from build123d import *

# Parameters (mm, degrees)
F1_DEPTH = 50
F2_DEPTH = 13
F4_DEPTH = 74.001
F5_R     = 1.25
F6_DEPTH = 15
F7_W     = 3
F7_H     = 10
F8_DEPTH = 8
F7_R     = 1.75
F9_DEPTH = 25


with BuildPart() as f1:
    # F0 (on Top) → F1 (new body)
    with BuildSketch(Plane.XY):
        Polygon((-17.5, 12), (-17.5, 0), (0, 0), (17.5, 0), (17.5, 12), (13.5, 12), (13.5, 8), (-13.5, 8), (-13.5, 12), align=None)
    extrude(amount=-F1_DEPTH)

    # F0 (on Top) → F2 (join)
    with BuildSketch(Plane.XY):
        with BuildLine():
            Line((-37, 0), (-37, -8))
            ThreePointArc((-37, -8), (-30, -15), (-23, -8))
            Line((-23, -8), (-23, 0))
            Line((-23, 0), (-17.5, 0))
            Line((-17.5, 0), (-17.5, 12))
            Line((-17.5, 12), (-37, 4))
            Line((-37, 4), (-37, 0))
        make_face()
        with BuildLine():
            Line((17.5, 12), (17.5, 0))
            Line((17.5, 0), (23, 0))
            Line((23, 0), (23, -8))
            ThreePointArc((23, -8), (30, -15), (37, -8))
            Line((37, -8), (37, 0))
            Line((37, 0), (37, 4))
            Line((37, 4), (17.5, 12))
        make_face()
    extrude(amount=-F2_DEPTH)

    # F3 (on face) → F4 (cut, through all)
    with BuildSketch(Plane(origin=(-37, 0, 0), x_dir=(0, -1, 0), z_dir=(-1, 0, 0))):
        Polygon((8, -11.267949), (8, -13), (15, -13), (15, -7.226497), align=None)
        Polygon((5, -13), (8, -13), (8, -11.267949), align=None)
    extrude(amount=-F4_DEPTH, mode=Mode.SUBTRACT)

    # F5 (on face) → F6 (cut)
    with BuildSketch(Plane(origin=(0, -6.879165, -11.915064), x_dir=(1, 0, 0), z_dir=(0, -0.5, -0.866025))):
        with Locations((-30, 3.377132)):
            Circle(F5_R)
        with Locations((30, 3.377132)):
            Circle(F5_R)
    extrude(amount=-F6_DEPTH, mode=Mode.SUBTRACT)

    # F7 (on face) → F8 (join)
    with BuildSketch(Plane.XZ):
        with BuildLine():
            Line((17.03, 0), (7.03, 0))
            Line((7.03, 0), (7.03, -10))
            Line((7.03, -10), (8.197224, -10))
            ThreePointArc((8.197224, -10), (10, -9.5), (11.802776, -10))
            Line((11.802776, -10), (17.03, -10))
            Line((17.03, -10), (17.03, 0))
        make_face()
        with BuildLine():
            Line((6.39, -1.259825), (6.39, -1))
            Line((6.39, -1), (6.39, -0.740175))
            ThreePointArc((6.39, -0.740175), (6.352771, -0.641268), (6.259565, -0.591457))
            ThreePointArc((6.259565, -0.591457), (6.101938, -0.557612), (5.951798, -0.498876))
            ThreePointArc((5.951798, -0.498876), (5.724361, -0.294149), (5.64, 0))
            Line((5.64, 0), (-0.36, 0))
            ThreePointArc((-0.36, 0), (-0.444361, -0.294149), (-0.671798, -0.498876))
            ThreePointArc((-0.671798, -0.498876), (-0.821938, -0.557612), (-0.979565, -0.591457))
            ThreePointArc((-0.979565, -0.591457), (-1.072771, -0.641268), (-1.11, -0.740175))
            Line((-1.11, -0.740175), (-1.11, -1))
            Line((-1.11, -1), (-1.11, -1.259825))
            ThreePointArc((-1.11, -1.259825), (-1.072771, -1.358732), (-0.979565, -1.408543))
            ThreePointArc((-0.979565, -1.408543), (-0.821938, -1.442388), (-0.671798, -1.501124))
            ThreePointArc((-0.671798, -1.501124), (-0.444361, -1.705851), (-0.36, -2))
            ThreePointArc((-0.36, -2), (-0.444361, -2.294149), (-0.671798, -2.498876))
            ThreePointArc((-0.671798, -2.498876), (-0.821938, -2.557612), (-0.979565, -2.591457))
            ThreePointArc((-0.979565, -2.591457), (-1.072771, -2.641268), (-1.11, -2.740175))
            Line((-1.11, -2.740175), (-1.11, -3))
            Line((-1.11, -3), (-1.11, -3.259825))
            ThreePointArc((-1.11, -3.259825), (-1.072771, -3.358732), (-0.979565, -3.408543))
            ThreePointArc((-0.979565, -3.408543), (-0.821938, -3.442388), (-0.671798, -3.501124))
            ThreePointArc((-0.671798, -3.501124), (-0.444361, -3.705851), (-0.36, -4))
            ThreePointArc((-0.36, -4), (-0.444361, -4.294149), (-0.671798, -4.498876))
            ThreePointArc((-0.671798, -4.498876), (-0.821938, -4.557612), (-0.979565, -4.591457))
            ThreePointArc((-0.979565, -4.591457), (-1.072771, -4.641268), (-1.11, -4.740175))
            Line((-1.11, -4.740175), (-1.11, -5))
            Line((-1.11, -5), (-1.11, -5.259825))
            ThreePointArc((-1.11, -5.259825), (-1.072771, -5.358732), (-0.979565, -5.408543))
            ThreePointArc((-0.979565, -5.408543), (-0.821938, -5.442388), (-0.671798, -5.501124))
            ThreePointArc((-0.671798, -5.501124), (-0.444361, -5.705851), (-0.36, -6))
            ThreePointArc((-0.36, -6), (-0.444361, -6.294149), (-0.671798, -6.498876))
            ThreePointArc((-0.671798, -6.498876), (-0.821938, -6.557612), (-0.979565, -6.591457))
            ThreePointArc((-0.979565, -6.591457), (-1.072771, -6.641268), (-1.11, -6.740175))
            Line((-1.11, -6.740175), (-1.11, -7))
            Line((-1.11, -7), (-1.11, -7.259825))
            ThreePointArc((-1.11, -7.259825), (-1.072771, -7.358732), (-0.979565, -7.408543))
            ThreePointArc((-0.979565, -7.408543), (-0.821938, -7.442388), (-0.671798, -7.501124))
            ThreePointArc((-0.671798, -7.501124), (-0.444361, -7.705851), (-0.36, -8))
            ThreePointArc((-0.36, -8), (-0.444361, -8.294149), (-0.671798, -8.498876))
            ThreePointArc((-0.671798, -8.498876), (-0.821938, -8.557612), (-0.979565, -8.591457))
            ThreePointArc((-0.979565, -8.591457), (-1.072771, -8.641268), (-1.11, -8.740175))
            Line((-1.11, -8.740175), (-1.11, -9))
            Line((-1.11, -9), (-1.11, -9.259825))
            ThreePointArc((-1.11, -9.259825), (-1.072771, -9.358732), (-0.979565, -9.408543))
            ThreePointArc((-0.979565, -9.408543), (-0.821938, -9.442388), (-0.671798, -9.501124))
            ThreePointArc((-0.671798, -9.501124), (-0.444361, -9.705851), (-0.36, -10))
            ThreePointArc((-0.36, -10), (2.64, -13), (5.64, -10))
            ThreePointArc((5.64, -10), (5.724361, -9.705851), (5.951798, -9.501124))
            ThreePointArc((5.951798, -9.501124), (6.101938, -9.442388), (6.259565, -9.408543))
            ThreePointArc((6.259565, -9.408543), (6.352771, -9.358732), (6.39, -9.259825))
            Line((6.39, -9.259825), (6.39, -9))
            Line((6.39, -9), (6.39, -8.740175))
            ThreePointArc((6.39, -8.740175), (6.352771, -8.641268), (6.259565, -8.591457))
            ThreePointArc((6.259565, -8.591457), (6.101938, -8.557612), (5.951798, -8.498876))
            ThreePointArc((5.951798, -8.498876), (5.724361, -8.294149), (5.64, -8))
            ThreePointArc((5.64, -8), (5.724361, -7.705851), (5.951798, -7.501124))
            ThreePointArc((5.951798, -7.501124), (6.101938, -7.442388), (6.259565, -7.408543))
            ThreePointArc((6.259565, -7.408543), (6.352771, -7.358732), (6.39, -7.259825))
            Line((6.39, -7.259825), (6.39, -7))
            Line((6.39, -7), (6.39, -6.740175))
            ThreePointArc((6.39, -6.740175), (6.352771, -6.641268), (6.259565, -6.591457))
            ThreePointArc((6.259565, -6.591457), (6.101938, -6.557612), (5.951798, -6.498876))
            ThreePointArc((5.951798, -6.498876), (5.724361, -6.294149), (5.64, -6))
            ThreePointArc((5.64, -6), (5.724361, -5.705851), (5.951798, -5.501124))
            ThreePointArc((5.951798, -5.501124), (6.101938, -5.442388), (6.259565, -5.408543))
            ThreePointArc((6.259565, -5.408543), (6.352771, -5.358732), (6.39, -5.259825))
            Line((6.39, -5.259825), (6.39, -5))
            Line((6.39, -5), (6.39, -4.740175))
            ThreePointArc((6.39, -4.740175), (6.352771, -4.641268), (6.259565, -4.591457))
            ThreePointArc((6.259565, -4.591457), (6.101938, -4.557612), (5.951798, -4.498876))
            ThreePointArc((5.951798, -4.498876), (5.724361, -4.294149), (5.64, -4))
            ThreePointArc((5.64, -4), (5.724361, -3.705851), (5.951798, -3.501124))
            ThreePointArc((5.951798, -3.501124), (6.101938, -3.442388), (6.259565, -3.408543))
            ThreePointArc((6.259565, -3.408543), (6.352771, -3.358732), (6.39, -3.259825))
            Line((6.39, -3.259825), (6.39, -3))
            Line((6.39, -3), (6.39, -2.740175))
            ThreePointArc((6.39, -2.740175), (6.352771, -2.641268), (6.259565, -2.591457))
            ThreePointArc((6.259565, -2.591457), (6.101938, -2.557612), (5.951798, -2.498876))
            ThreePointArc((5.951798, -2.498876), (5.724361, -2.294149), (5.64, -2))
            ThreePointArc((5.64, -2), (5.724361, -1.705851), (5.951798, -1.501124))
            ThreePointArc((5.951798, -1.501124), (6.101938, -1.442388), (6.259565, -1.408543))
            ThreePointArc((6.259565, -1.408543), (6.352771, -1.358732), (6.39, -1.259825))
        make_face()
        with Locations((-3.25, -5)):
            Rectangle(F7_W, F7_H)
    extrude(amount=F8_DEPTH)

    # F7 (on face) → F9 (cut)
    with BuildSketch(Plane.XZ):
        with Locations((-10, -13)):
            Circle(F7_R)
        with Locations((10, -13)):
            Circle(F7_R)
        with Locations((10, -33)):
            Circle(F7_R)
        with Locations((-10, -33)):
            Circle(F7_R)
    extrude(amount=-F9_DEPTH, mode=Mode.SUBTRACT)


solid = f1.part
Design review of the part built by this model. Coordinates are the model's own, in mm. A direction names the side the tool comes from. Coordinates: 2 decimals unless noted, no trailing zeros. Loops run counter-clockwise (first coordinate to the right, second up) from the corner with the lowest first, then second, coordinate; pieces in that order, holes last. Notation, with made-up numbers: (26.25, -33.75) -> (44.25, -33.75) arc R18 ccw to (44.25, -8.75) -> close; hole circle Ø11 at (8, 54.5). An arc over 180 degrees is marked (long way). Use a Markdown table: item, result. Add a question column.
Item 1: The part is to be moulded in two halves that separate along Z. For faces 1 (the flat face through (-1, 2, 0)), 2 (the cylindrical face through (10.9, 3.9, -31.5)), 3 (the cylindrical face through (30.58, -5.72, -5.37)), 4 (the flat face through (-17.5, 6, -31)), say which applies: +Z half, -Z half, draft (parallel to the pull), parting line (faces both ways), or undercut.
Item 2: We need section A-A, the plane z = -33. Write out the cut boundary in (x, y).
Item 3: We need section D-D, the plane x = 30. Write out the cut boundary in (y, z), and give its area (3 significant figures).
Item 4: Machinability: for faces 5 (the flat face through (7.03, -4, -5)), 6 (the flat face through (0, 8, -25)), 7 (the cylindrical face through (2.6, -3.9, -13)), 8 (the flat face through (0, 5, -50)), which of the approach directions +Z, -Z, +X, -X, +Y, -Y give a long, thin tool a straight path to every point of the face, cutting with its end or side? Answer none if there is none.
Item 5: We need section C-C, the plane y = -12.5. Write out the cut boundary in (x, z), and give its area (3 significant figures).
Item 6: Wall thickness on L1, parallel to Z at x = 10, y = 3.5; L2, parallel to Z at x = -22.5, y = 4.5; L3, parallel to X at y = 7.25, z = -16.5: over which ranges is each line inside the solid? List them lowest first. Write a range as from..to.
Item 7: We need section B-B, the plane x = -10. Write out the cut boundary in (y, z), and give its area (3 significant figures).
Item 8: Clearance check with flat-ended pins moving along their axes: P1, Ø10, axis at y = -1.5, z = -29, coming from the +X side; P2, Ø6, axis at x = 14, z = -29, coming from the -Y side; P3, Ø3, axis at x = 10, z = -35, coming from the +Y side. State where each tip first meets the part, or that it passes through.
Numbers:
| question | item | result |
|---|---|---|
| 1 | face 1 | +Z half |
| 1 | face 2 | undercut |
| 1 | face 3 | undercut |
| 1 | face 4 | draft |
| 2 | outline | (-17.5, 0) -> (-11.75, 0) -> (-11.75, 8) -> (-13.5, 8) -> (-13.5, 12) -> (-17.5, 12) -> close; (-8.25, 0) -> (8.25, 0) -> (8.25, 8) -> (-8.25, 8) -> close; (11.75, 0) -> (17.5, 0) -> (17.5, 12) -> (13.5, 12) -> (13.5, 8) -> (11.75, 8) -> close |
| 3 | outline | (-15, -7.23) -> (-10.89, -9.6) -> (-5.34, 0) -> (-15, 0) -> close; (-8.72, -10.85) -> (-5, -13) -> (6.87, -13) -> (6.87, 0) -> (-2.46, 0) -> close |
| 3 | area | 226 mm^2 |
| 4 | face 5 | +Z, -Z, -Y |
| 4 | face 6 | +Z, -Z, +Y |
| 4 | face 7 | -Z, -Y |
| 4 | face 8 | -Z, +X, -X, +Y, -Y |
| 5 | outline | (-35.36, -8.67) -> (-24.64, -8.67) -> (-24.64, 0) -> (-35.36, 0) -> close; (24.64, -8.67) -> (35.36, -8.67) -> (35.36, 0) -> (24.64, 0) -> close |
| 5 | area | 186 mm^2 |
| 6 | L1 | z = -50..-34.75, -31.25..-14.75, -11.25..0 |
| 6 | L2 | z = -13..0 |
| 6 | L3 | x = -17.5..17.5 |
| 7 | outline | (0, -50) -> (8, -50) -> (8, -34.75) -> (0, -34.75) -> close; (0, -31.25) -> (8, -31.25) -> (8, -14.75) -> (0, -14.75) -> close; (0, -11.25) -> (8, -11.25) -> (8, 0) -> (0, 0) -> close |
| 7 | area | 344 mm^2 |
| 8 | P1 | stops at x = 17.5 |
| 8 | P2 | stops at y = 0 |
| 8 | P3 | stops at y = 8 |
